Check sheet for the modelled part. Datum: model origin and axes. Units: mm. Face numbers are marked on the shaded views. Round coordinates to 2 decimals unless told otherwise and drop trailing zeros. Loops run counter-clockwise (first coordinate to the right, second up) from the corner with the lowest first, then second, coordinate; pieces in that order, holes last. Notation, with made-up numbers: (-14, 30) -> (-4, 30) arc R15 ccw to (-4, 50) -> close; hole circle Ø3 at (-33, -0.75). An arc over 180 degrees is marked (long way). One line per item, written item: value. Start each with the question number.
1. Material ranges on L1, parallel to Z at x = 28.5, y = 2.25; L2, parallel to Y at x = 13, z = -2.1; L3, parallel to Y at x = 21, z = -38.2, recorded low to high.
2. Go/stop test with flat-tipped pins: pin 1 (1.2 mm diameter, centred on x = 5, y = 2, fed in from +Z); pin 2 (20 mm diameter, centred on x = 28, z = -14, fed in from +Y); pin 3 (1.6 mm diameter, centred on x = 6.5, y = 10, fed in from +Z). Record where each tip stops, or that it passes through.
3. Cross-section at A-A on y = 12.75. Record the cut outline in (x, z).
4. Release check for a two-part mould opening along Z. For the marked faces 1, 2 and 3 record: +Z half, -Z half, draft (parallel to the pull), parting line (faces both ways), or undercut.
from build123d import *

# Parameters (mm, degrees)
SKETCH1_W                = 40
SKETCH1_H                = 40
BOSS_EXTRUDE1_DEPTH      = 20
SKETCH2_R                = 4
BOSS_EXTRUDE2_DEPTH      = 2
BOSS_EXTRUDE2_DEPTH_BACK = 43
SKETCH3_R                = 10
BOSS_EXTRUDE3_DEPTH      = 3
SKETCH4_R                = 10
BOSS_EXTRUDE4_DEPTH      = 4
SKETCH5_R                = 1
CUT_EXTRUDE1_DEPTH       = 5
SKETCH6_R                = 1
CUT_EXTRUDE2_DEPTH       = 5


with BuildPart() as part:
    # Sketch1 → Boss-Extrude1 (new body)
    with BuildSketch(Plane(origin=(0, 0, 0), x_dir=(1, 0, 0), z_dir=(0, 1, 0))):
        with Locations((20, 20)):
            Rectangle(SKETCH1_W, SKETCH1_H)
    extrude(amount=BOSS_EXTRUDE1_DEPTH)

    # Sketch2 → Boss-Extrude2 (add, two sides)
    with BuildSketch(Plane.XY) as boss_extrude2_sk:
        with Locations((29.985325212, 10.020295376)):
            Circle(SKETCH2_R)
    extrude(amount=BOSS_EXTRUDE2_DEPTH)
    extrude(boss_extrude2_sk.sketch, amount=-BOSS_EXTRUDE2_DEPTH_BACK)

    # Sketch3 → Boss-Extrude3 (add)
    with BuildSketch(Plane.XY.offset(2)):
        with Locations((29.985325212, 10.020295376)):
            Circle(SKETCH3_R)
    extrude(amount=BOSS_EXTRUDE3_DEPTH)

    # Sketch4 → Boss-Extrude4 (add)
    with BuildSketch(Plane(origin=(0, 0, -43), x_dir=(-1, 0, 0), z_dir=(0, 0, -1))):
        with Locations((-29.985325212, 10.020295376)):
            Circle(SKETCH4_R)
    extrude(amount=BOSS_EXTRUDE4_DEPTH)

    # Sketch5 → Cut-Extrude1 (cut)
    with BuildSketch(Plane(origin=(0, 0, -40), x_dir=(-1, 0, 0), z_dir=(0, 0, -1))):
        with Locations((-5, 18)):
            Circle(SKETCH5_R)
        with Locations((-5, 2)):
            Circle(SKETCH5_R)
        with Locations((-21, 2)):
            Circle(SKETCH5_R)
        with Locations((-21, 18)):
            Circle(SKETCH5_R)
    extrude(amount=-CUT_EXTRUDE1_DEPTH, mode=Mode.SUBTRACT)

    # Sketch6 → Cut-Extrude2 (cut)
    with BuildSketch(Plane.XY):
        with Locations((13, 16.5)):
            Circle(SKETCH6_R)
        with Locations((6.5, 10)):
            Circle(SKETCH6_R)
        with Locations((13, 3.5)):
            Circle(SKETCH6_R)
        with Locations((19.5, 10)):
            Circle(SKETCH6_R)
    extrude(amount=-CUT_EXTRUDE2_DEPTH, mode=Mode.SUBTRACT)


solid = part.part
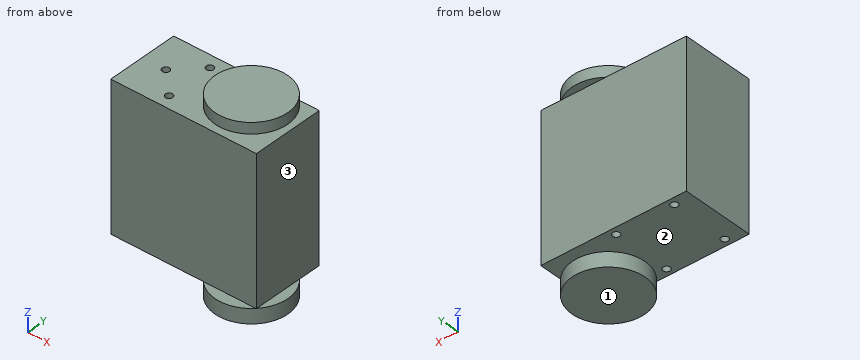
Taken from the geometry:
1. L1: z = -47 to -43, -40 to 0, 2 to 5
1. L2: y = 0 to 2.5, 4.5 to 15.5, 17.5 to 20
1. L3: y = 0 to 1, 3 to 17, 19 to 20
2. pin 1: stops at z = 0
2. pin 2: stops at y = 20
2. pin 3: stops at z = -5
3. outline: (0, -40) -> (27.06, -40) -> (27.06, -43) -> (20.37, -43) -> (20.37, -47) -> (39.61, -47) -> (39.61, -43) -> (32.91, -43) -> (32.91, -40) -> (40, -40) -> (40, 0) -> (32.91, 0) -> (32.91, 2) -> (39.61, 2) -> (39.61, 5) -> (20.37, 5) -> (20.37, 2) -> (27.06, 2) -> (27.06, 0) -> (0, 0) -> close
4. face 1: -Z half
4. face 2: undercut
4. face 3: draft
